```python
from build123d import *

# Parameters (mm, degrees)
F0_W     = 25.4
F0_H     = 25.4
F1_DEPTH = 25.4
F2_W     = 19.05
F2_H     = 19.05
F3_DEPTH = 19.05
F4_W     = 19.05
F4_H     = 19.05
F4_W_2   = 12.7
F4_H_2   = 12.7
F5_DEPTH = 6.35
F6_R     = 2.54


with BuildPart() as f1:
    # F0 (on Top) → F1 (new body)
    with BuildSketch(Plane.XY):
        with Locations((12.7, -12.7)):
            Rectangle(F0_W, F0_H)
    extrude(amount=F1_DEPTH)

    # F2 (on face) → F3 (cut)
    with BuildSketch(Plane(origin=(0, 0, 0), x_dir=(1, 0, 0), z_dir=(0, 0, -1))):
        with Locations((12.7, 12.7)):
            Rectangle(F2_W, F2_H)
    extrude(amount=-F3_DEPTH, mode=Mode.SUBTRACT)

    # F4 (on face) → F5 (join)
    with BuildSketch(Plane.XY.offset(25.4)):
        with Locations((12.7, -12.7)):
            Rectangle(F4_W, F4_H)
        with Locations((12.7, -12.7)):
            Rectangle(F4_W_2, F4_H_2, mode=Mode.SUBTRACT)
    extrude(amount=F5_DEPTH)

    # F6
    f6_edges = [f1.edges().sort_by_distance(p)[0] for p in [
        (0, 0, 12.7),
        (0, -25.4, 12.7),
        (25.4, 0, 12.7),
        (3.175, -3.175, 28.575),
        (3.175, -22.225, 28.575),
        (22.225, -3.175, 28.575),
        (22.225, -22.225, 28.575),
        (25.4, -25.4, 12.7),
    ]]
    fillet(f6_edges, radius=F6_R)


solid = f1.part
```
Read the model definition and answer for the solid it produces. Units are mm, in the model's axes. A direction names the side the tool comes from. Round coordinates to 2 decimals unless told otherwise and drop trailing zeros. Write each loop counter-clockwise with the first axis right and the second up, starting at its lowest first coordinate (ties: lowest second). Pieces come first, ordered by that corner, then holes. Notation, with made-up numbers: M 58,25 L 80,25 A16 cw 80,47 Z; hole C 88,-6.75 d2. An arc over 180 degrees is marked long. One line per item, written item: value.
Q1. Flat-ended cylindrical pins translate along their axes: pin 1 Ø3 at (x, z) = (12, 28) entering from +Y (3 decimals); pin 2 Ø7 at (y, z) = (-11, 29) entering from -X (3 decimals); pin 3 Ø1.9 at (y, z) = (-15, 27) entering from +X (3 decimals); pin 4 Ø15 at (x, y) = (9, -16) entering from -Z. Find the tip coordinate at first contact, or state that the pin passes through.
Data:
pin 1: y = -3.175
pin 2: x = 3.175
pin 3: x = 22.225
pin 4: z = 0
Q2. Straight lines are drawn through the part: line 1 (X direction, y = -15.25, z = 30.5) (3 decimals); line 2 (X direction, y = -21.5, z = 8.5) (3 decimals); line 3 (Y direction, x = 14.75, z = 1.5) (3 decimals). For each, find the intervals that lie inside material, in ascending order. Write a range as [from, to].
Data:
line 1: [3.175, 6.35], [19.05, 22.225]
line 2: [0, 3.175], [22.225, 25.4]
line 3: [-25.4, -22.225], [-3.175, 0]
Q3. Find section B-B on x = 13.25. Write down the section's boundary in (y, z) (3 decimals).
Data:
outline: M -25.4,0 L -22.225,0 L -22.225,19.05 L -3.175,19.05 L -3.175,0 L 0,0 L 0,25.4 L -3.175,25.4 L -3.175,31.75 L -6.35,31.75 L -6.35,25.4 L -19.05,25.4 L -19.05,31.75 L -22.225,31.75 L -22.225,25.4 L -25.4,25.4 Z
Q4. Which of the six approach directions +Z, -Z, +X, -X, +Y, -Y give full straight-line access (tool end or side, diameter ignored) to faces 4 (the flat face through (13, -3.175, 29)), 5 (the cylindrical face through (3.94, -21.5, 28.62)), 6 (the flat face through (13, -13, 25.4)), 7 (the cylindrical face through (3.94, -3.9, 28.62)), 8 (the flat face through (13, -13, 19.05))?
Data:
face 4: +Z, +X, -X, +Y
face 5: +Z, -X, -Y
face 6: +Z
face 7: +Z, -X, +Y
face 8: -Z
Q5. Find section D-D on y = -4.5. Write down the section's boundary in (x, z) (3 decimals), plus the area to 3 significant figures.
Data:
outline: M 0,0 L 3.175,0 L 3.175,19.05 L 22.225,19.05 L 22.225,0 L 25.4,0 L 25.4,25.4 L 21.916,25.4 L 21.916,31.75 L 3.484,31.75 L 3.484,25.4 L 0,25.4 Z
area: 399 mm2
Q6. Find section A-A on z = 15. Write down the section's boundary in (x, y) (3 decimals).
Data:
outline: M 0,-22.86 A2.54 ccw 2.54,-25.4 L 22.86,-25.4 A2.54 ccw 25.4,-22.86 L 25.4,-2.54 A2.54 ccw 22.86,0 L 2.54,0 A2.54 ccw 0,-2.54 Z; hole M 3.175,-22.225 L 22.225,-22.225 L 22.225,-3.175 L 3.175,-3.175 Z
Q7. Find section C-C on y = -11.5. Write down the section's boundary in (x, z) (3 decimals), plus the area to 3 significant figures.
Data:
outline: M 0,0 L 3.175,0 L 3.175,19.05 L 22.225,19.05 L 22.225,0 L 25.4,0 L 25.4,25.4 L 22.225,25.4 L 22.225,31.75 L 19.05,31.75 L 19.05,25.4 L 6.35,25.4 L 6.35,31.75 L 3.175,31.75 L 3.175,25.4 L 0,25.4 Z
area: 323 mm2
Q8. For a pull along X with two mould halves and no side action, classify faces 1 (the flat face through (3.175, -13, 29)), 2 (the cylindrical face through (21.46, -21.5, 28.62)), 3 (the flat face through (13, -19.05, 29)) as +X half, -X half, draft (parallel to the pull), parting line (faces both ways), or undercut.
Data:
face 1: -X half
face 2: +X half
face 3: undercut
